```python
from build123d import *

# Parameters (mm, degrees)
SKETCH4_R          = 9.525
CUT_EXTRUDE1_DEPTH = 123.803155497


with BuildPart() as part:
    # Sketch2 → Revolve1 (revolve)
    with BuildSketch(Plane.XY, mode=Mode.PRIVATE) as revolve1_sk:
        Polygon((0, 16.611620209), (-82.55, 16.611620209), (-82.55, 7.086620209), (-69.85, 7.086620209), (-69.85, -11.963379791), (-82.55, -11.963379791), (-82.55, -21.488379791), (0, -21.488379791), align=None)
    revolve(revolve1_sk.sketch.rotate(Axis((0, 36.56493994, 0), (0, -1, 0)), 270), axis=Axis((0, 36.56493994, 0), (0, -1, 0)))

    # Sketch4 → Cut-Extrude1 (cut, through all)
    with BuildSketch(Plane(origin=(0, 16.611620209, 0), x_dir=(1, 0, 0), z_dir=(0, 1, 0))):
        with Locations(Location((0, 0, 0), (0, 0, 270))):
            Circle(SKETCH4_R)
    extrude(amount=-CUT_EXTRUDE1_DEPTH, mode=Mode.SUBTRACT)


solid = part.part
```
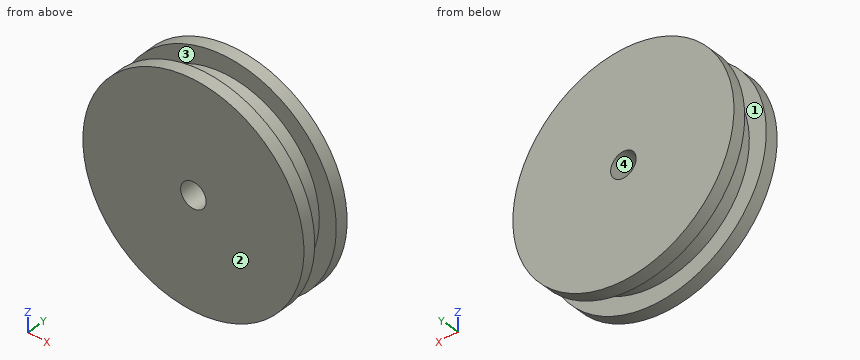
Verification items for the finished model (mm, model axes). Face numbers are marked on the shaded views. A direction names the side the tool comes from. Give positions to 0.01 mm unless a question says otherwise; leave off trailing zeros. Write each loop counter-clockwise with the first axis right and the second up, starting at its lowest first coordinate (ties: lowest second). Pieces come first, ordered by that corner, then holes. Notation, with made-up numbers: (-25.75, -36) - (19.25, -36) arc R33 ccw to (19.25, -8) - close; hole circle Ø1 at (0, 74.5). An arc over 180 degrees is marked (long way). Put each result on its own line as item: value.
Q1. Section check C-C on y = -3. Record the cut outline in (x, z) (3 decimals), and give its area (3 significant figures).
Result:
outline: circle Ø139.7 at (0, 0); hole circle Ø19.05 at (0, 0)
area: 15,000 mm2
Q2. Section check D-D on x = 25.5. Record the cut outline in (y, z).
Result:
outline: (-21.49, -78.51) - (-11.96, -78.51) - (-11.96, -65.03) - (7.09, -65.03) - (7.09, -78.51) - (16.61, -78.51) - (16.61, 78.51) - (7.09, 78.51) - (7.09, 65.03) - (-11.96, 65.03) - (-11.96, 78.51) - (-21.49, 78.51) - close
Q3. Scan lines: probe 1 along X at (y, z) = (-1, 0) (3 decimals); probe 2 along Y at (x, z) = (69, -15.5); probe 3 along Z at (x, y) = (-50, 5). Record each from-to range of solid material in increasing order. Write a range as from..to.
Result:
probe 1: -69.85..-9.525, 9.525..69.85
probe 2: -21.49..-11.96, 7.09..16.61
probe 3: -48.78..48.78
Q4. Set-up check for the marked faces 1 and 2: record each of +Z, -Z, +X, -X, +Y, -Y from which the full face is reachable in a straight line by a thin tool's end or side.
Result:
face 1: none
face 2: +Z, -Z, +X, -X, -Y
Q5. Depth check by flat-ended pin: P1, Ø3, axis at x = 25, y = 9.5, coming from the -Z side; P2, Ø2, axis at x = -39.5, y = -5.5, coming from the +Z side; P3, Ø25, axis at x = 0, z = 0, coming from the -Y side; P4, Ø10, axis at y = -17.5, z = 51, coming from the -X side. Enter the tip coordinate at first touch or a pass-through.
Result:
P1: z = -79.13
P2: z = 58.28
P3: y = -21.49
P4: x = -68.55
Q6. Section check B-B on z = 0. Record the cut outline in (x, y) (3 decimals), and give its area (3 significant figures).
Result:
outline: (-82.55, -21.488) - (-9.525, -21.488) - (-9.525, 16.612) - (-82.55, 16.612) - (-82.55, 7.087) - (-69.85, 7.087) - (-69.85, -11.963) - (-82.55, -11.963) - close; (9.525, -21.488) - (82.55, -21.488) - (82.55, -11.963) - (69.85, -11.963) - (69.85, 7.087) - (82.55, 7.087) - (82.55, 16.612) - (9.525, 16.612) - close
area: 5,080 mm2
Q7. Mould release check, pull along X, two halves, no side actions. Record for the marked faces 3 and 4: released by +X, released by -X, zero draft, split by the parting line, or undercut.
Result:
face 3: zero draft
face 4: undercut
Q8. Section check A-A on x = 0. Record the cut outline in (y, z) (3 decimals).
Result:
outline: (-21.488, -82.55) - (-11.963, -82.55) - (-11.963, -69.85) - (7.087, -69.85) - (7.087, -82.55) - (16.612, -82.55) - (16.612, -9.525) - (-21.488, -9.525) - close; (-21.488, 9.525) - (16.612, 9.525) - (16.612, 82.55) - (7.087, 82.55) - (7.087, 69.85) - (-11.963, 69.85) - (-11.963, 82.55) - (-21.488, 82.55) - close
